```python
from build123d import *

# Parameters (mm, degrees)
SKETCH1_R           = 1.525
SKETCH1_R_2         = 1.5
BOSS_EXTRUDE1_DEPTH = 6
FILLET1_SIZE        = 10
FILLET1_SIZE_2      = 30


with BuildPart() as part:
    # Sketch1 → Boss-Extrude1 (new body)
    with BuildSketch(Plane(origin=(0, 0, 0), x_dir=(1, 0, 0), z_dir=(0, 1, 0))):
        Polygon((500, 0), (0, 0), (0, -165), (150, -165), (150, -315), (0, -315), (0, -480), (500, -480), align=None)
        with Locations(Location((10, -474, 0), (0, 0, 270))):
            Circle(SKETCH1_R, mode=Mode.SUBTRACT)
        with Locations(Location((490, -474, 0), (0, 0, 270))):
            Circle(SKETCH1_R_2, mode=Mode.SUBTRACT)
        with Locations(Location((10, -6, 0), (0, 0, 270))):
            Circle(SKETCH1_R_2, mode=Mode.SUBTRACT)
        with Locations(Location((490, -6, 0), (0, 0, 270))):
            Circle(SKETCH1_R_2, mode=Mode.SUBTRACT)
    extrude(amount=BOSS_EXTRUDE1_DEPTH)

    # Fillet1
    # an asymmetric fillet: 30, 10 mm, written as the material it adds along each edge
    with BuildSketch(Plane(origin=(150, 0, 315), x_dir=(0, 0, -1), z_dir=(0, 1, 0)), Plane(origin=(150, 0, 165), x_dir=(-1, 0, 0), z_dir=(0, 1, 0))) as fillet1_piece_1:
        with BuildLine():
            Bezier((FILLET1_SIZE, 0), (0, 0), (0, FILLET1_SIZE_2), weights=[1, 0.707106781, 1])
            Line((0, FILLET1_SIZE_2), (0, 0))
            Line((0, 0), (FILLET1_SIZE, 0))
        make_face()
    extrude(amount=6)
    # an asymmetric fillet: 30, 10 mm, written as the material it takes off along each edge
    with BuildSketch(Plane(origin=(0, -75, 165), x_dir=(0, 0, -1), z_dir=(0, 1, 0)), Plane(origin=(0, -75, 315), x_dir=(1, 0, 0), z_dir=(0, 1, 0))) as fillet1_2_piece_1:
        with BuildLine():
            Bezier((FILLET1_SIZE, 0), (0, 0), (0, -FILLET1_SIZE_2), weights=[1, 0.707106781, 1])
            Line((0, -FILLET1_SIZE_2), (0, 0))
            Line((0, 0), (FILLET1_SIZE, 0))
        make_face()
    extrude(amount=156, mode=Mode.SUBTRACT)


solid = part.part
```
Part model, mm, in its own coordinate system. Round coordinates to 2 decimals unless told otherwise and drop trailing zeros. Loops run counter-clockwise (first coordinate to the right, second up) from the corner with the lowest first, then second, coordinate; pieces in that order, holes last.
Item 1: Cut at A-A, the plane y = 3. State how many separate pieces and enclosed holes the cut face has, then the cut area to 3 significant figures.
Item 2: Cut at B-B, the plane z = 298.5. Give the cut face in (x, y), then the cut area to 3 significant figures.
Item 3: Drill centre lines: line 1 (X direction, y = 4.2, z = 6); line 2 (Z direction, x = 490, y = 1.6); line 3 (X direction, y = 5.25, z = 257.5). Where is each one in solid material? Low to high.
A:
1. separate pieces: 1
1. enclosed holes: 4
1. area: 217,000 mm2
2. outline: (150, 0) - (500, 0) - (500, 6) - (150, 6) - close
2. area: 2,100 mm2
3. line 1: x = 0 to 8.5, 11.5 to 488.5, 491.5 to 500
3. line 2: z = 0 to 4.5, 7.5 to 472.5, 475.5 to 480
3. line 3: x = 150 to 500
